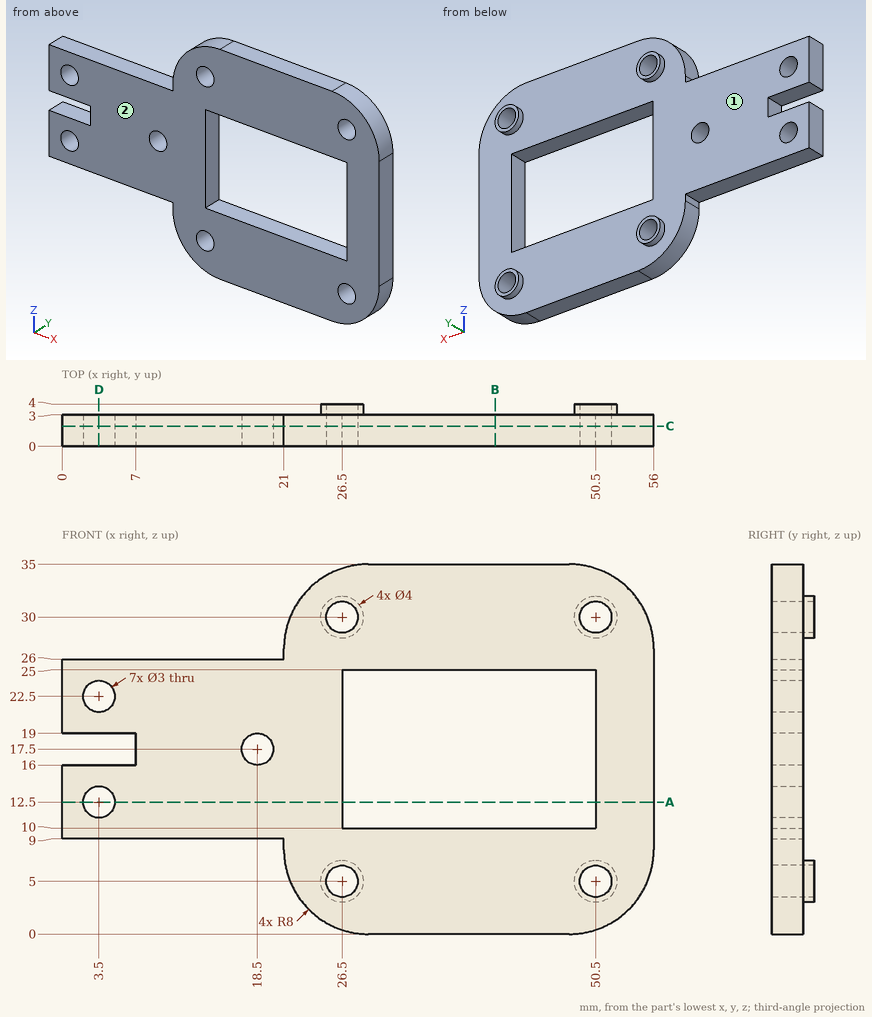
Source: three-view drawing plus pictorial views. Frame: mm from the lowest corner of the part. A direction names the side the tool comes from. Coordinates: 2 decimals unless noted, no trailing zeros. Write each loop counter-clockwise with the first axis right and the second up, starting at its lowest first coordinate (ties: lowest second). Pieces come first, ordered by that corner, then holes. Notation, with made-up numbers: (54.5, -22.75) -> (101.5, -22.75) arc R33 cw to (101.5, 10.25) -> close; hole circle Ø9 at (83.5, 69.25). An arc over 180 degrees is marked (long way). Answer as a JSON object with one key per item and string values.
1. First-contact query: P1, Ø1.5, axis at x = 4, y = 1, coming from the -Z side; P2, Ø0.5, axis at y = 1, z = 26.5, coming from the -X side; P3, Ø2, axis at x = 14.5, y = 3, coming from the +Z side; P4, Ø2.5, axis at x = 18.5, z = 17.5, coming from the -Y side. Flat tips, straight axial feed; report the tip coordinate or a pass-through.
Result set:
{"P1": "stops at z = 9", "P2": "stops at x = 21", "P3": "stops at z = 26", "P4": "passes through"}
2. Section A-A on z = 12.5. Return the cut outline in (x, y), then the cut area to 3 significant figures.
Result set:
{"outline": "(0, 0) -> (2, 0) -> (2, 3) -> (0, 3) -> close; (5, 0) -> (26.5, 0) -> (26.5, 3) -> (5, 3) -> close; (50.5, 0) -> (56, 0) -> (56, 3) -> (50.5, 3) -> close", "area": "87.0 mm2"}
3. Access query for the marked faces 1 and 2. Directions: +Z, -Z, +X, -X, +Y, -Y. A direction counts if a zero-diameter tool reaches every point of the face in a straight line with its end or side. Return the directions, or none.
Result set:
{"face 1": "+Y", "face 2": "+Z, -Z, +X, -X, -Y"}
4. Material intervals for line 1 (X direction, y = 0.75, z = 12.5); line 2 (X direction, y = 3.15, z = 30); line 3 (X direction, y = 1.5, z = 5), sorted ascending. Write a range as from..to.
Result set:
{"line 1": "x = 0..2, 5..26.5, 50.5..56", "line 2": "x = 24.5..25, 28..28.5, 48.5..49, 52..52.5", "line 3": "x = 21.58..25, 28..49, 52..55.42"}
5. Section C-C on y = 1.9. Count the separate pieces of the cut face and the enclosed holes in it, then the cut area to 3 significant figures.
Result set:
{"separate pieces": "1", "enclosed holes": "8", "area": "1,100 mm2"}
6. Section B-B on x = 41. Return the cut outline in (y, z), then the cut area to 3 significant figures.
Result set:
{"outline": "(0, 0) -> (3, 0) -> (3, 10) -> (0, 10) -> close; (0, 25) -> (3, 25) -> (3, 35) -> (0, 35) -> close", "area": "60.0 mm2"}
7. Section D-D on x = 3.5. Return the cut outline in (y, z), then the cut area to 3 significant figures.
Result set:
{"outline": "(0, 9) -> (3, 9) -> (3, 11) -> (0, 11) -> close; (0, 14) -> (3, 14) -> (3, 16) -> (0, 16) -> close; (0, 19) -> (3, 19) -> (3, 21) -> (0, 21) -> close; (0, 24) -> (3, 24) -> (3, 26) -> (0, 26) -> close", "area": "24.0 mm2"}
